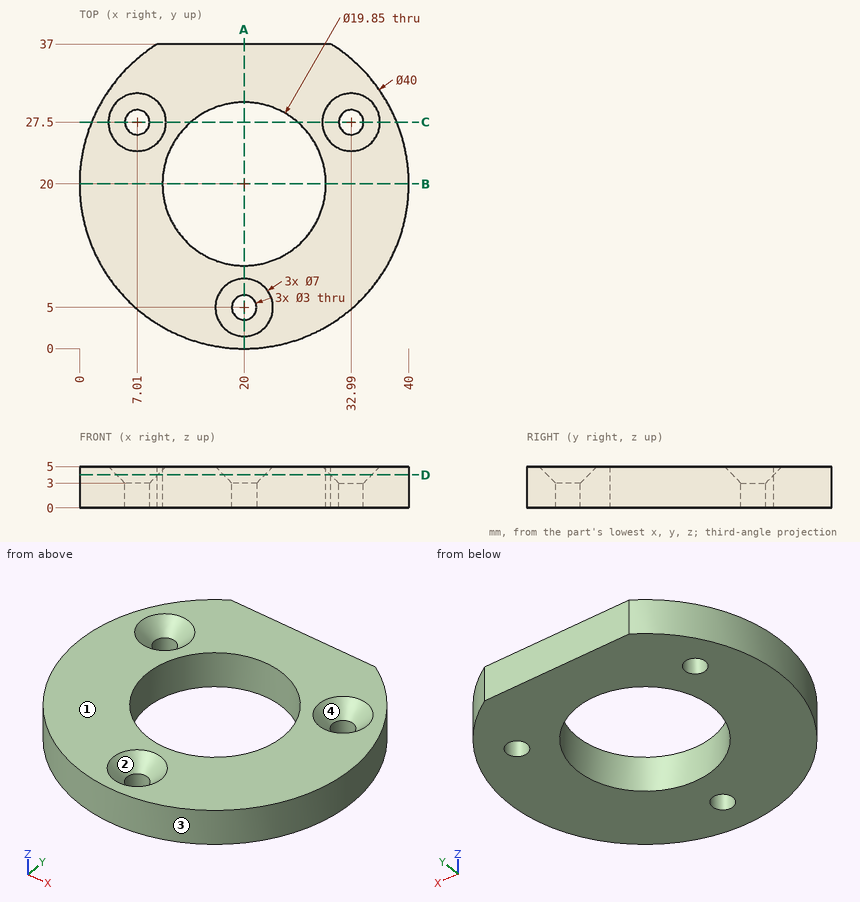
Answer from the drawing. Dimensions are ordinates in mm from the lowest x, y and z of the part. Give positions to 0.01 mm unless a question says otherwise; leave off trailing zeros. Loops run counter-clockwise (first coordinate to the right, second up) from the corner with the lowest first, then second, coordinate; pieces in that order, holes last.
Item 1: Find the intervals of material crossed by line 1 along Y through (x, z) = (20, 2.15) (1 decimal); line 2 along X through (y, z) = (3, 2.35) (1 decimal); line 3 along Y through (x, z) = (32.5, 1.8), in increasing order.
Item 2: The part is cut by section D-D (z = 4). Give the number of separate pieces and of enclosed holes in the cut face.
Item 3: The mould has two halves that part along X. Classify the marked faces 1, 2, 3 and 4: released by +X, released by -X, zero draft, split by the parting line, or undercut.
Item 4: The part is cut by section A-A (x = 20). Write down the section's boundary in (y, z) (1 decimal).
Item 5: Each of these flat-tipped pins is pushed along its axis until it touches: pin 1 Ø4 at (x, y) = (7.01, 27.5) entering from +Z; pin 2 Ø2.5 at (x, y) = (20, 5) entering from -Z; pin 3 Ø1 at (x, z) = (28.5, 1.5) entering from -Y. Where does it stop, or does it pass through?
Item 6: The part is cut by section C-C (y = 27.5). Write down the section's boundary in (x, z).
Item 7: The part is cut by section B-B (y = 20). Write down the section's boundary in (x, z) (1 decimal), and give its area (3 significant figures).
Taken from the geometry:
1. line 1: y = 0 to 3.5, 6.5 to 10.1, 29.9 to 37
1. line 2: x = 9.5 to 30.5
1. line 3: y = 4.39 to 26.08, 28.92 to 35.61
2. separate pieces: 1
2. enclosed holes: 4
3. face 1: zero draft
3. face 2: undercut
3. face 3: split by the parting line
3. face 4: undercut
4. outline: (0, 0) - (3.5, 0) - (3.5, 3) - (1.5, 5) - (0, 5) - close; (6.5, 0) - (10.1, 0) - (10.1, 5) - (8.5, 5) - (6.5, 3) - close; (29.9, 0) - (37, 0) - (37, 5) - (29.9, 5) - close
5. pin 1: stops at z = 3.5
5. pin 2: passes through
5. pin 3: stops at y = 1.67
6. outline: (1.46, 0) - (5.51, 0) - (5.51, 3) - (3.51, 5) - (1.46, 5) - close; (8.51, 0) - (13.5, 0) - (13.5, 5) - (10.51, 5) - (8.51, 3) - close; (26.5, 0) - (31.49, 0) - (31.49, 3) - (29.49, 5) - (26.5, 5) - close; (34.49, 0) - (38.54, 0) - (38.54, 5) - (36.49, 5) - (34.49, 3) - close
7. outline: (0, 0) - (10.1, 0) - (10.1, 5) - (0, 5) - close; (29.9, 0) - (40, 0) - (40, 5) - (29.9, 5) - close
7. area: 101 mm2
